from build123d import *

# Parameters (mm, degrees)
F0_R     = 101.6
F1_DEPTH = 38.1
F2_R     = 95.25
F2_R_2   = 44.45
F3_DEPTH = 25.4
F4_R     = 95.25
F4_R_2   = 44.45
F5_DEPTH = 25.4
F7_D     = 19.05
F8_SIZE  = 0.762


with BuildPart() as f1:
    # F0 (on Front) → F1 (new body, symmetric)
    with BuildSketch(Plane.XZ):
        Circle(F0_R)
    extrude(amount=F1_DEPTH, both=True)

    # F2 (on face) → F3 (cut)
    with BuildSketch(Plane.XZ.offset(38.1)):
        Circle(F2_R)
        Circle(F2_R_2, mode=Mode.SUBTRACT)
    extrude(amount=-F3_DEPTH, mode=Mode.SUBTRACT)

    # F4 (on face) → F5 (cut)
    with BuildSketch(Plane(origin=(0, 38.1, 0), x_dir=(-1, 0, 0), z_dir=(0, 1, 0))):
        Circle(F4_R)
        Circle(F4_R_2, mode=Mode.SUBTRACT)
    extrude(amount=-F5_DEPTH, mode=Mode.SUBTRACT)

    # F7 (through all)
    with Locations(Plane.XZ.offset(38.1)):
        with Locations((0, 0)):
            Hole(F7_D / 2)

    # F8
    f8_edges = [f1.edges().sort_by_distance(p)[0] for p in [
        (-44.45, -38.1, 0),
        (-95.25, -38.1, 0),
        (-101.6, -38.1, 0),
        (44.45, 38.1, 0),
        (95.25, 38.1, 0),
        (-101.6, 38.1, 0),
        (-9.525, 38.1, 0),
        (-9.525, -38.1, 0),
    ]]
    chamfer(f8_edges, length=F8_SIZE)


solid = f1.part
Can you work these out from the model? Positions are in its coordinate system, mm. A direction names the side the tool comes from. Coordinates: 2 decimals unless noted, no trailing zeros. Write each loop counter-clockwise with the first axis right and the second up, starting at its lowest first coordinate (ties: lowest second). Pieces come first, ordered by that corner, then holes. Notation, with made-up numbers: (22, 65) -> (47, 65) arc R14 ccw to (47, 77) -> close; hole circle Ø11 at (76, 26.25). An arc over 180 degrees is marked (long way). Write each question's results on one line, items separated by ' | '. Start each with the question number.
Q1. Imagine slicing it at B-B (y = -8). Write out the boundary of the cut face in (x, z) (3 decimals), then the cut area to 3 significant figures.
Q2. If I drill on probe 1 along Z at (x, y) = (0, -20.5) (3 decimals); probe 2 along Z at (x, y) = (-16.5, 27.5); probe 3 along X at (y, z) = (24, -5), over which ranges is the centre line in solid material (lowest first)?
Q3. I'm going to push flat-ended pins straight in: pin 1 (1 mm diameter, centred on y = -24.5, z = 27.5, fed in from -X); pin 2 (1 mm diameter, centred on x = -33, y = -30, fed in from -Z); pin 3 (8 mm diameter, centred on x = -75, z = 40.5, fed in from -Y). Where does each tip first touch, or does it pass through?
Q4. On a 3-axis mill with a long thin cutter (end or side, diameter ignored), from which of +Z, -Z, +X, -X, +Y, -Y can I reach the whole of each face in a straight line? I mean faces 4 (the face through (41, -12.7, -20)), 5 (the face through (-41, 12.7, -20)), 6 (the face through (89, -38.1, -37)). Say none if no direction works.
Q5. We'd pull the mould along Z, two halves only. Please class faces 1 (the face through (9, -38.1, -9)), 2 (the face through (-22.025, -0.523, -99.184)), 3 (the face through (7.559, 0.523, -5.796)): +Z half, -Z half, draft (parallel to the pull), parting line (faces both ways), or undercut.
Q6. Imagine slicing it at A-A (y = 31). Write out the boundary of the cut face in (x, z) (3 decimals), then the cut area to 3 significant figures.
Taken from the geometry:
1) outline: circle Ø203.2 at (0, 0); hole circle Ø19.05 at (0, 0) | area: 32,100 mm^2
2) probe 1: z = -101.6 to -95.25, -44.45 to -9.525, 9.525 to 44.45, 95.25 to 101.6 | probe 2: z = -100.25 to -93.81, -41.27 to 41.27, 93.81 to 100.25 | probe 3: x = -101.48 to -95.12, -44.17 to -8.11, 8.11 to 44.17, 95.12 to 101.48
3) pin 1: stops at x = -97.95 | pin 2: stops at z = -96.26 | pin 3: stops at y = -12.7
4) face 4: -Y | face 5: +Y | face 6: +Z, -Z, +X, -X, -Y
5) face 1: draft | face 2: parting line | face 3: undercut
6) outline: circle Ø203.2 at (0, 0); circle Ø88.9 at (0, 0); hole circle Ø190.5 at (0, 0); hole circle Ø19.05 at (0, 0) | area: 9,850 mm^2
